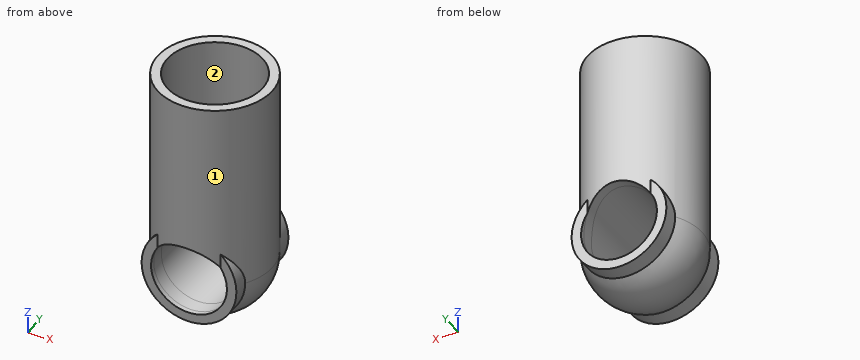
from build123d import *

# Parameters (mm, degrees)
SKETCH_1_R               = 12
SKETCH_1_R_2             = 10
EXTRUDE_1_DEPTH          = 40
SKETCH_3_R               = 10
SKETCH_3_R_2             = 8
EXTRUDE_2_DEPTH          = 10
CUT_EXTRUDE_1_DEPTH      = 44.451122112
CUT_EXTRUDE_1_DEPTH_BACK = 44.451122112
SKETCH_4_R               = 8


with BuildPart() as part:
    # 草图1 → 凸台-拉伸1 (new body)
    with BuildSketch(Plane.XY):
        Circle(SKETCH_1_R)
        Circle(SKETCH_1_R_2, mode=Mode.SUBTRACT)
    extrude(amount=EXTRUDE_1_DEPTH)

    # 草图2 → 旋转1 (revolve)
    with BuildSketch(Plane(origin=(0, 0, 0), x_dir=(1, 0, 0), z_dir=(0, 1, 0))):
        with BuildLine():
            Line((-12, 0), (-10, 0))
            ThreePointArc((-10, 0), (-7.071067812, 7.071067812), (0, 10))
            Line((0, 10), (0, 12))
            ThreePointArc((0, 12), (-8.485281374, 8.485281374), (-12, 0))
        make_face()
    revolve(axis=Axis((0, 0, -10), (0, 0, 1)))

    # 草图3 → 凸台-拉伸2 (add, symmetric)
    with BuildSketch(Plane(origin=(0, 0, 0), x_dir=(1, 0, 0), z_dir=(0, 1, 0))):
        Circle(SKETCH_3_R)
        with Locations(Location((0, 0, 0), (0, 0, 180))):
            Circle(SKETCH_3_R_2, mode=Mode.SUBTRACT)
    extrude(amount=EXTRUDE_2_DEPTH, both=True)

    # 草图4 → 切除-拉伸1 (cut, two sides: drawn at the far end of the back side and taken through both)
    with BuildSketch(Plane(origin=(0, 0, 0), x_dir=(1, 0, 0), z_dir=(0, 1, 0)).offset(-CUT_EXTRUDE_1_DEPTH_BACK)):
        with Locations(Location((0, 0, 0), (0, 0, 213.987843581))):
            Circle(SKETCH_4_R)
    extrude(amount=CUT_EXTRUDE_1_DEPTH + CUT_EXTRUDE_1_DEPTH_BACK, mode=Mode.SUBTRACT)


solid = part.part
Read the model definition and answer for the solid it produces. Units are mm, in the model's axes. Face numbers are marked on the shaded views. Give positions to 0.01 mm unless a question says otherwise; leave off trailing zeros. Loops run counter-clockwise (first coordinate to the right, second up) from the corner with the lowest first, then second, coordinate; pieces in that order, holes last. Notation, with made-up numbers: (-5.75, -19.5) -> (36.25, -19.5) arc R4 ccw to (36.25, -12.5) -> close; hole circle Ø3 at (73.5, 54). An arc over 180 degrees is marked (long way). Use a Markdown table: item, result.
Q1. Find the intervals of material crossed by line 1 along Y through (x, z) = (0, 22.5); line 2 along X through (y, z) = (8.25, 0), in increasing order.
Solved:
| item | result |
|---|---|
| line 1 | y = -12 to -10, 10 to 12 |
| line 2 | x = -10 to -8, 8 to 10 |
Q2. Section D-D, the plane x = 5.5 is taken. Determine the outline of the cut face in (y, z), then the cut area to 3 significant figures.
Solved:
| item | result |
|---|---|
| outline | (-10.67, 5.81) -> (10.67, 5.81) -> (10.67, 40) -> (8.35, 40) -> (8.35, 8.35) -> (-8.35, 8.35) -> (-8.35, 40) -> (-10.67, 40) -> close; (-10, -8.35) -> (-6.63, -8.35) arc R10.67 ccw to (6.63, -8.35) -> (10, -8.35) -> (10, -5.81) -> (-10, -5.81) -> close |
| area | 272 mm^2 |
Q3. Section B-B, the plane x = 0 is taken. Determine the outline of the cut face in (y, z).
Solved:
| item | result |
|---|---|
| outline | (-12, 8) -> (12, 8) -> (12, 40) -> (10, 40) -> (10, 10) -> (-10, 10) -> (-10, 40) -> (-12, 40) -> close; (-10, -10) -> (-6.63, -10) arc R12 ccw to (6.63, -10) -> (10, -10) -> (10, -8) -> (-10, -8) -> close |
Q4. Section A-A, the plane y = 0 is taken. Determine the outline of the cut face in (x, z), then the cut area to 3 significant figures.
Solved:
| item | result |
|---|---|
| outline | (-12, 0) arc R12 ccw to (12, 0) -> (12, 40) -> (10, 40) -> (10, 0) arc R10 ccw to (-10, 0) -> (-10, 40) -> (-12, 40) -> close; hole circle Ø16 at (0, 0) |
| area | 342 mm^2 |
Q5. Determine the mould class of the marked faces 1 and 2 for opening direction X: pulls with the +X half, pulls with the -X half, needs draft (parallel to the pull), parting line crosses it, or undercut.
Solved:
| item | result |
|---|---|
| face 1 | parting line crosses it |
| face 2 | undercut |
Q6. Section C-C, the plane z = -7 is taken. Determine the outline of the cut face in (x, y), then the cut area to 3 significant figures.
Solved:
| item | result |
|---|---|
| outline | (-7.14, -10) -> (-3.87, -10) -> (-3.87, 10) -> (-7.14, 10) -> (-7.14, 6.63) arc R9.75 ccw to (-7.14, -6.63) -> close; (3.87, -10) -> (7.14, -10) -> (7.14, -6.63) arc R9.75 ccw to (7.14, 6.63) -> (7.14, 10) -> (3.87, 10) -> close |
| area | 178 mm^2 |
Q7. Each of these flat-tipped pins is pushed along its axis until it touches: pin 1 (12 mm diameter, centred on y = 8.5, z = -2, fed in from +X); pin 2 (6 mm diameter, centred on x = 4, z = 11.5, fed in from +Y); pin 3 (1 mm diameter, centred on y = -6, z = 18, fed in from -X); pin 4 (4 mm diameter, centred on x = -6.5, y = 6.5, fed in from +Z). Where does it stop, or does it pass through?
Solved:
| item | result |
|---|---|
| pin 1 | stops at x = 11.68 |
| pin 2 | stops at y = 11.96 |
| pin 3 | stops at x = -10.67 |
| pin 4 | stops at z = 40 |
